Verification items for the finished model (mm, model axes). Round coordinates to 2 decimals unless told otherwise and drop trailing zeros. Write each loop counter-clockwise with the first axis right and the second up, starting at its lowest first coordinate (ties: lowest second). Pieces come first, ordered by that corner, then holes. Notation, with made-up numbers: (63.5, -22) - (119.5, -22) arc R14 ccw to (119.5, -17) - close; hole circle Ø8 at (-27.5, -1.5). An arc over 180 degrees is marked (long way). Answer as a JSON object with one key per item and string values.
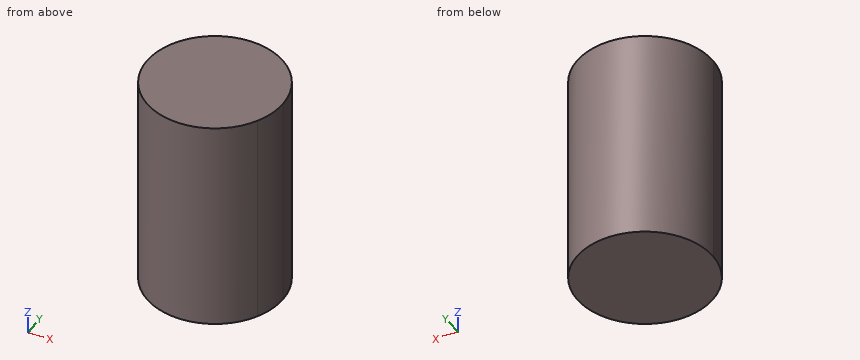
Autodesk Inventor part; units mm, degrees
ref_plane "Work Plane1" through (-26.797, -37.3063, 85.979) normal (0, 0, -1) x (0, 1, 0)
ref_plane "YZ Plane" through (0, 0, 0) normal (1, 0, 0) x (0, 1, 0)
ref_plane "XZ Plane" through (0, 0, 0) normal (0, 1, 0) x (-1, 0, 0)
ref_plane "Work Plane1" through (-26.797, -37.3063, 85.979) normal (0, 0, -1) x (0, 1, 0)
sketch "Sketch1" plane through (0, 0, 0) normal (0, 0, 1) x (1, 0, 0)
  arc A0 (-23.9286, -16.5336) -> (-20.447, -28.194) centre (-20.447, -21.844) ccw
  line L0 (-20.447, -28.194) -> (20.447, -28.194)
  arc A1 (20.447, -28.194) -> (23.9286, -16.5336) centre (20.447, -21.844) ccw
  arc A2 (23.4121, -14.4336) -> (23.9286, -16.5336) centre (24.799, -15.206) ccw
  arc A3 (23.4121, -14.4336) -> (26.797, -1.397) centre (0, -1.397) ccw
  line L1 (26.797, -1.397) -> (26.797, 19.05)
  arc A4 (26.797, 19.05) -> (20.447, 25.4) centre (20.447, 19.05) ccw
  line L2 (20.447, 25.4) -> (-20.447, 25.4)
  arc A5 (-20.447, 25.4) -> (-26.797, 19.05) centre (-20.447, 19.05) ccw
  line L3 (-26.797, 19.05) -> (-26.797, -1.397)
  arc A6 (-26.797, -1.397) -> (-23.4121, -14.4336) centre (0, -1.397) ccw
  arc A7 (-23.9286, -16.5336) -> (-23.4121, -14.4336) centre (-24.799, -15.206) ccw
  circle A8 centre (0, -1.397) radius 26.797
  point P0 (0, 0)
  dimension "d0" = 53.594
extrude "Extrusion1" add sketch "Sketch1" along normal blind 85.2932 contours A6 A8 A3
properties part number "Pneumatics_VIAIR_00090_03"
1. Cross-section at A-A (z = 67.5). Record the boundary of the cut face in (x, y), plus the area to 3 significant figures.
Completed:
{"outline": "(-26.8, -1.4) arc R26.8 ccw to (-23.41, -14.43) arc R26.8 ccw to (23.41, -14.43) arc R26.8 ccw to (26.8, -1.4) arc R26.8 ccw to start", "area": "2,260 mm^2"}
2. Go/stop test with flat-tipped pins: pin 1 (2 mm diameter, centred on y = 14, z = 11.5, fed in from +X); pin 2 (12 mm diameter, centred on x = -8, z = 37.5, fed in from -Y); pin 3 (1 mm diameter, centred on y = -14.5, z = 68.5, fed in from -X). Record where each tip stops, or that it passes through.
Completed:
{"pin 1": "stops at x = 22.6", "pin 2": "stops at y = -28.12", "pin 3": "stops at x = -23.65"}
3. Cross-section at B-B (x = -10). Record the boundary of the cut face in (y, z).
Completed:
{"outline": "(-26.26, 0) - (23.46, 0) - (23.46, 85.29) - (-26.26, 85.29) - close"}
4. Material ranges on probe 1 along Y at (x, z) = (1, 74); probe 2 along X at (y, z) = (8.5, 54); probe 3 along Y at (x, z) = (5.5, 48), recorded low to high. Write a range as from..to.
Completed:
{"probe 1": "y = -28.18..25.38", "probe 2": "x = -24.9..24.9", "probe 3": "y = -27.62..24.83"}
